For this review, take the finished solid that the model builds, in its own axes (mm). A direction names the side the tool comes from. Round coordinates to 2 decimals unless told otherwise and drop trailing zeros. Order: outer loops, then holes, each group sorted by start corner. A loop starts at its lowest first (then second) coordinate and runs counter-clockwise, first axis right, second up. Notation, with made-up numbers: (7, 47.25) - (21, 47.25) arc R10 cw to (21, 54.25) - close; hole circle Ø6 at (80, -9). An arc over 180 degrees is marked (long way). One line per question, with ' | ' between items.
```python
from build123d import *

# Parameters (mm, degrees)
EXTRUDE_1_DEPTH     = 150
SHELL_1_T           = -2
SKETCH_2_R          = 1.7
SKETCH_2_W          = 21
SKETCH_2_H          = 42.435234345
CUT_EXTRUDE_1_DEPTH = 150
SKETCH_3_W          = 11.907125669
SKETCH_3_H          = 29.749118518
CUT_EXTRUDE_2_DEPTH = 10
FILLET_1_R          = 2
FILLET_2_R          = 2
FILLET_3_R          = 2
FILLET_4_R          = 2
SKETCH_4_R          = 1.5
CUT_EXTRUDE_3_DEPTH = 7
SKETCH_5_R          = 1.5
CUT_EXTRUDE_4_DEPTH = 7


with BuildPart() as part:
    # 草图1 → 凸台-拉伸1 (new body)
    with BuildSketch(Plane.XY):
        with BuildLine():
            Line((-28.318229719, 20.413532085), (-28.318229719, -29.586467915))
            ThreePointArc((-28.318229719, -29.586467915), (-25.38929753, -36.657535727), (-18.318229719, -39.586467915))
            Line((-18.318229719, -39.586467915), (31.681770281, -39.586467915))
            ThreePointArc((31.681770281, -39.586467915), (38.752838093, -36.657535727), (41.681770281, -29.586467915))
            Line((41.681770281, -29.586467915), (41.681770281, 20.413532085))
            ThreePointArc((41.681770281, 20.413532085), (38.752838093, 27.484599896), (31.681770281, 30.413532085))
            Line((31.681770281, 30.413532085), (-18.318229719, 30.413532085))
            ThreePointArc((-18.318229719, 30.413532085), (-25.38929753, 27.484599896), (-28.318229719, 20.413532085))
        make_face()
    extrude(amount=EXTRUDE_1_DEPTH)

    # 抽壳1
    shell_1_openings = [part.faces().sort_by_distance(p)[0] for p in [
        (6.681770281, -4.586467915, 150),
    ]]
    offset(amount=SHELL_1_T, openings=shell_1_openings, kind=Kind.INTERSECTION)

    # 草图2 → 切除-拉伸1 (cut)
    with BuildSketch(Plane(origin=(0, 0, 0), x_dir=(-1, 0, 0), z_dir=(0, 0, -1))):
        with Locations((16.070445421, 20.123532085)):
            Circle(SKETCH_2_R)
        with Locations(Location((6.070445421, 20.123532085, 0), (0, 0, 180))):
            Circle(SKETCH_2_R)
        with Locations(Location((16.070445421, -29.296467915, 0), (0, 0, 180))):
            Circle(SKETCH_2_R)
        with Locations((6.070445421, -29.296467915)):
            Circle(SKETCH_2_R)
        with Locations((11.070445421, -4.586467916)):
            Rectangle(SKETCH_2_W, SKETCH_2_H)
    extrude(amount=-CUT_EXTRUDE_1_DEPTH, mode=Mode.SUBTRACT)

    # 草图3 → 切除-拉伸2 (cut)
    with BuildSketch(Plane(origin=(0, 0, 0), x_dir=(-1, 0, 0), z_dir=(0, 0, -1))):
        with Locations((-21.578307669, -5.268329048)):
            Rectangle(SKETCH_3_W, SKETCH_3_H)
    extrude(amount=-CUT_EXTRUDE_2_DEPTH, mode=Mode.SUBTRACT)

    # 圆角1
    fillet_1_edges = [part.edges().sort_by_distance(p)[0] for p in [
        (15.624744835, 9.606230211, 1),
    ]]
    fillet(fillet_1_edges, radius=FILLET_1_R)

    # 圆角2
    fillet_2_edges = [part.edges().sort_by_distance(p)[0] for p in [
        (15.624744835, -20.142888307, 1),
    ]]
    fillet(fillet_2_edges, radius=FILLET_2_R)

    # 圆角3
    fillet_3_edges = [part.edges().sort_by_distance(p)[0] for p in [
        (27.531870504, -20.142888307, 1),
    ]]
    fillet(fillet_3_edges, radius=FILLET_3_R)

    # 圆角4
    fillet_4_edges = [part.edges().sort_by_distance(p)[0] for p in [
        (27.531870504, 9.606230211, 1),
    ]]
    fillet(fillet_4_edges, radius=FILLET_4_R)

    # 草图4 → 切除-拉伸3 (cut)
    with BuildSketch(Plane.ZY.offset(-39.681770281)):
        with Locations((147, -22.586467915)):
            Circle(SKETCH_4_R)
    extrude(amount=-CUT_EXTRUDE_3_DEPTH, mode=Mode.SUBTRACT)

    # 草图5 → 切除-拉伸4 (cut)
    with BuildSketch(Plane(origin=(-26.318229719, 0, 0), x_dir=(0, 0, -1), z_dir=(1, 0, 0))):
        with Locations((-147, 13.413532085)):
            Circle(SKETCH_5_R)
    extrude(amount=-CUT_EXTRUDE_4_DEPTH, mode=Mode.SUBTRACT)


solid = part.part
```
(1) For probe 1 along Y at (x, z) = (19, 83); probe 2 along X at (y, z) = (8, 70); probe 3 along Z at (x, y) = (38, 1), list the stretches that pass through material, from the lowest coordinate up. Write a range as [from, to].
Output values:
probe 1: [-39.59, -37.59], [28.41, 30.41] | probe 2: [-28.32, -26.32], [39.68, 41.68] | probe 3: [0, 2]
(2) Insertion check: pin 1 (20 mm diameter, centred on x = 16, y = 4.5, fed in from +Z); pin 2 (3 mm diameter, centred on x = -6.07, y = 20.12, fed in from -Z). Each pin has a flat end and moves straight along its axis. Give the tip position at first contact, or say it passes through.
Output values:
pin 1: z = 2 | pin 2: through
(3) We need section B-B on x = -2.5. State the section outline as (y, z) points.
Output values:
outline: (-39.59, 0) - (-25.8, 0) - (-25.8, 2) - (-37.59, 2) - (-37.59, 150) - (-39.59, 150) - close; (16.63, 0) - (30.41, 0) - (30.41, 150) - (28.41, 150) - (28.41, 2) - (16.63, 2) - close
(4) For faces 1 (the cylindrical face through (40.668, -21.573, 145.894)), 2 (the flat face through (6, -4, 2)), 3 (the flat face through (-28.318, -4, 74)), list the 3-axis set-ups (+Z, -Z, +X, -X, +Y, -Y) from which the entire face can be reached by the end or side of a thin tool; tool diameter is ignored.
Output values:
face 1: +X | face 2: +Z | face 3: +Z, -Z, -X, +Y, -Y
(5) We need section A-A on z = 123. State the section outline as (x, y) points, plus the area to 3 significant figures.
Output values:
outline: (-28.32, -29.59) arc R10 ccw to (-18.32, -39.59) - (31.68, -39.59) arc R10 ccw to (41.68, -29.59) - (41.68, 20.41) arc R10 ccw to (31.68, 30.41) - (-18.32, 30.41) arc R10 ccw to (-28.32, 20.41) - close; hole (-26.32, -29.59) arc R8 ccw to (-18.32, -37.59) - (31.68, -37.59) arc R8 ccw to (39.68, -29.59) - (39.68, 20.41) arc R8 ccw to (31.68, 28.41) - (-18.32, 28.41) arc R8 ccw to (-26.32, 20.41) - close | area: 513 mm^2
(6) We need section C-C on z = 147. State the section outline as (x, y) points.
Output values:
outline: (-28.32, -29.59) arc R10 ccw to (-18.32, -39.59) - (31.68, -39.59) arc R10 ccw to (41.68, -29.59) - (41.68, -24.09) - (39.68, -24.09) - (39.68, -29.59) arc R8 cw to (31.68, -37.59) - (-18.32, -37.59) arc R8 cw to (-26.32, -29.59) - (-26.32, 11.91) - (-28.32, 11.91) - close; (-28.32, 14.91) - (-26.32, 14.91) - (-26.32, 20.41) arc R8 cw to (-18.32, 28.41) - (31.68, 28.41) arc R8 cw to (39.68, 20.41) - (39.68, -21.09) - (41.68, -21.09) - (41.68, 20.41) arc R10 ccw to (31.68, 30.41) - (-18.32, 30.41) arc R10 ccw to (-28.32, 20.41) - close
(7) Mouldability with a two-part tool opening along Y and no side actions: class faces 4 (the cylindrical face through (-14.72, 19.09, 0.99)), 5 (the cylindrical face through (38.83, 27.406, 73.95)), 6 (the flat face through (7, 29, 150)) as released by +Y, released by -Y, zero draft, split by the parting line, or undercut.
Output values:
face 4: undercut | face 5: released by +Y | face 6: zero draft
